from build123d import *

# Parameters (mm, degrees)
CROQUIS1_W              = 379
CROQUIS1_H              = 316
SALIENTE_EXTRUIR1_DEPTH = 180
VACIADO1_T              = -8
CROQUIS2_R              = 35
CORTAR_EXTRUIR4_DEPTH   = 20
CROQUIS4_R              = 45
CROQUIS4_R_2            = 40
SALIENTE_EXTRUIR4_DEPTH = 10
CROQUIS6_R              = 55
CORTAR_EXTRUIR6_DEPTH   = 10
CROQUIS7_R              = 24
CROQUIS7_R_2            = 21
SALIENTE_EXTRUIR9_DEPTH = 8


with BuildPart() as part:
    # Croquis1 → Saliente-Extruir1 (new body)
    with BuildSketch(Plane.XY):
        Rectangle(CROQUIS1_W, CROQUIS1_H)
    extrude(amount=SALIENTE_EXTRUIR1_DEPTH)

    # Vaciado1
    vaciado1_openings = [part.faces().sort_by_distance(p)[0] for p in [
        (0, 0, 180),
    ]]
    offset(amount=VACIADO1_T, openings=vaciado1_openings, kind=Kind.INTERSECTION)

    # Croquis2 → Cortar-Extruir4 (cut)
    with BuildSketch(Plane.ZY.offset(189.5)):
        with Locations((90, 58)):
            Circle(CROQUIS2_R)
    extrude(amount=-CORTAR_EXTRUIR4_DEPTH, mode=Mode.SUBTRACT)

    # Croquis4 → Saliente-Extruir4 (add)
    with BuildSketch(Plane(origin=(-181.5, 0, 0), x_dir=(0, 0, -1), z_dir=(1, 0, 0))):
        with Locations((-90, 58)):
            Circle(CROQUIS4_R)
        with Locations((-90, 58)):
            Circle(CROQUIS4_R_2, mode=Mode.SUBTRACT)
    extrude(amount=SALIENTE_EXTRUIR4_DEPTH)

    # Croquis6 → Cortar-Extruir6 (cut)
    with BuildSketch(Plane(origin=(189.5, 0, 0), x_dir=(0, 0, -1), z_dir=(1, 0, 0))):
        with Locations((-90, 58)):
            Circle(CROQUIS6_R)
    extrude(amount=-CORTAR_EXTRUIR6_DEPTH, mode=Mode.SUBTRACT)

    # Croquis7 → Saliente-Extruir9 (add)
    with BuildSketch(Plane.XY.offset(8)):
        with Locations(Location((0, -53, 0), (0, 0, 180))):
            Circle(CROQUIS7_R)
        with Locations((0, -53)):
            Circle(CROQUIS7_R_2, mode=Mode.SUBTRACT)
    extrude(amount=SALIENTE_EXTRUIR9_DEPTH)


solid = part.part
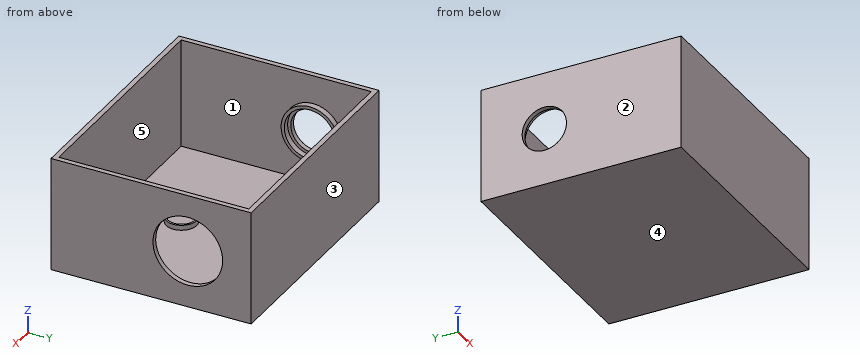
Input: part model. Units: mm. Frame: model coordinates. Face numbers are marked on the shaded views. A direction names the side the tool comes from. Give positions to 0.01 mm unless a question says otherwise; leave off trailing zeros. Order: outer loops, then holes, each group sorted by start corner. A loop starts at its lowest first (then second) coordinate and runs counter-clockwise, first axis right, second up. Notation, with made-up numbers: (15.25, -8) - (34.25, -8) arc R25 ccw to (34.25, 13) - close; hole circle Ø2 at (71.5, 57.25). An arc over 180 degrees is marked (long way). Answer as a JSON object with one key per item and string values. Group by question number.
Q1. Line query: probe 1 along Y at (x, z) = (0, 11); probe 2 along Y at (x, z) = (-185.75, 90); probe 3 along X at (y, z) = (-141, 43.5). Output: solid intervals per line, ascending.
Q2. Cut plane A-A, the plane y = 58. Output: boundary loops of the cut face in (x, z), then the cut area to 3 significant figures.
Q3. Set-up query: the marked faces 4 and 5. Return all of +Z, -Z, +X, -X, +Y, -Y with unobstructed straight access to the full face (end or side cutting, diameter ignored); none if empty.
Q4. Cut plane D-D, the plane x = 0. Output: boundary loops of the cut face in (y, z), then the cut area to 3 significant figures.
Q5. Cut plane B-B, the plane z = 25. Output: boundary loops of the cut face in (x, y).
Q6. First-contact query: pin 1 Ø3 at (x, y) = (80.5, -100.5) entering from +Z; pin 2 Ø6 at (y, z) = (52, 130.5) entering from +X. Flat tips, straight axial feed; report the tip coordinate or a pass-through.
Q7. Mould query, pull axis X, two halves, no side actions, for the marked faces 1, 2 and 3. Classes: pulls with the +X half, pulls with the -X half, needs draft (parallel to the pull), parting line crosses it, or undercut.
Q8. Cut plane C-C, the plane z = 90. Output: boundary loops of the cut face in (x, y), then the cut area to 3 significant figures.
Results:
{
 "1": {"probe 1": "-158 to -150, -77 to -74, -32 to -29, 150 to 158", "probe 2": "-158 to 23, 93 to 158", "probe 3": "-189.5 to -181.5, 181.5 to 189.5"},
 "2": {"outline": "(-189.5, 0) - (189.5, 0) - (189.5, 35) - (181.5, 35) - (181.5, 8) - (-181.5, 8) - (-181.5, 45) - (-171.5, 45) - (-171.5, 50) - (-181.5, 50) - (-181.5, 55) - (-189.5, 55) - close; (-189.5, 125) - (-181.5, 125) - (-181.5, 130) - (-171.5, 130) - (-171.5, 135) - (-181.5, 135) - (-181.5, 180) - (-189.5, 180) - close; (181.5, 145) - (189.5, 145) - (189.5, 180) - (181.5, 180) - close", "area": "4,440 mm^2"},
 "3": {"face 4": "-Z, +X, -X, +Y, -Y", "face 5": "+Z"},
 "4": {"outline": "(-158, 0) - (158, 0) - (158, 180) - (150, 180) - (150, 8) - (-29, 8) - (-29, 16) - (-32, 16) - (-32, 8) - (-74, 8) - (-74, 16) - (-77, 16) - (-77, 8) - (-150, 8) - (-150, 180) - (-158, 180) - close", "area": "5,330 mm^2"},
 "5": {"outline": "(-189.5, -158) - (189.5, -158) - (189.5, 158) - (-189.5, 158) - close; hole (-181.5, -150) - (181.5, -150) - (181.5, 150) - (-181.5, 150) - close"},
 "6": {"pin 1": "z = 8", "pin 2": "x = -171.5"},
 "7": {"face 1": "undercut", "face 2": "pulls with the -X half", "face 3": "needs draft"},
 "8": {"outline": "(-189.5, -158) - (189.5, -158) - (189.5, 3) - (181.5, 3) - (181.5, -150) - (-181.5, -150) - (-181.5, 13) - (-171.5, 13) - (-171.5, 18) - (-181.5, 18) - (-181.5, 23) - (-189.5, 23) - close; (-189.5, 93) - (-181.5, 93) - (-181.5, 98) - (-171.5, 98) - (-171.5, 103) - (-181.5, 103) - (-181.5, 150) - (181.5, 150) - (181.5, 113) - (189.5, 113) - (189.5, 158) - (-189.5, 158) - close", "area": "9,520 mm^2"}
}
